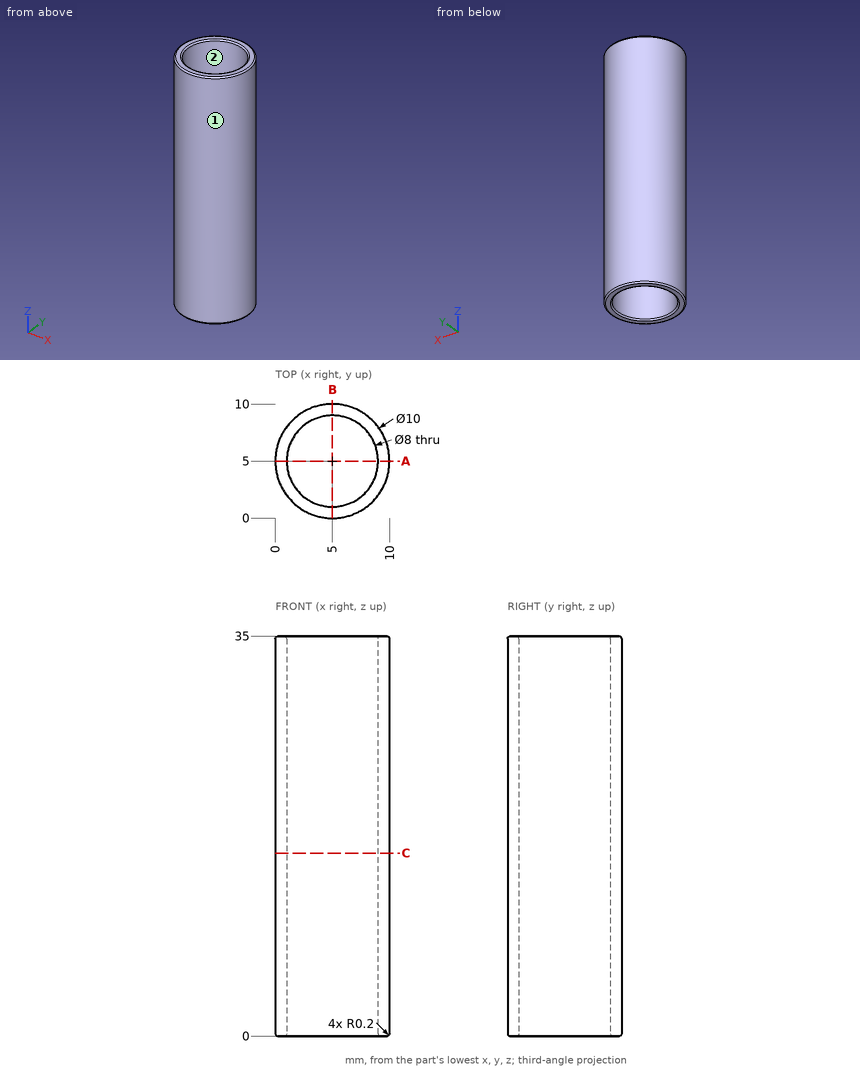
Verification items for this drawing (mm, ordinates from the low corner). Coordinates: 2 decimals unless noted, no trailing zeros. Loops run counter-clockwise (first coordinate to the right, second up) from the corner with the lowest first, then second, coordinate; pieces in that order, holes last.
Item 1: Thickness scan on line 1 (Y direction, x = 5, z = 20.5); line 2 (X direction, y = 5.25, z = 18.5); line 3 (Y direction, x = 8.5, z = 6). Record the ranges inside material, lowest first.
Item 2: Go/stop test with flat-tipped pins: pin 1 Ø6 at (x, y) = (6.5, 9) entering from -Z; pin 2 Ø3 at (x, z) = (2.5, 5.5) entering from -Y; pin 3 Ø1.5 at (y, z) = (7.5, 30) entering from -X; pin 4 Ø1 at (x, z) = (9, 8) entering from -Y. Record where each tip stops, or that it passes through.
Item 3: Sectioned sample at A-A, the plane y = 5. Record the boundary of the cut face in (x, z), then the cut area to 3 significant figures.
Item 4: Sectioned sample at C-C, the plane z = 16. Record the boundary of the cut face in (x, y), then the cut area to 3 significant figures.
Item 5: Release check for a two-part mould opening along Y. For the marked faces 1 and 2 record: released by +Y, released by -Y, zero draft, split by the parting line, or undercut.
Check result:
1. line 1: y = 0 to 1, 9 to 10
1. line 2: x = 0.01 to 1.01, 8.99 to 9.99
1. line 3: y = 1.43 to 3.06, 6.94 to 8.57
2. pin 1: stops at z = 0
2. pin 2: stops at y = 0.1
2. pin 3: stops at x = 0.32
2. pin 4: stops at y = 1.43
3. outline: (0, 0.2) arc R0.2 ccw to (0.2, 0) - (0.8, 0) arc R0.2 ccw to (1, 0.2) - (1, 34.8) arc R0.2 ccw to (0.8, 35) - (0.2, 35) arc R0.2 ccw to (0, 34.8) - close; (9, 0.2) arc R0.2 ccw to (9.2, 0) - (9.8, 0) arc R0.2 ccw to (10, 0.2) - (10, 34.8) arc R0.2 ccw to (9.8, 35) - (9.2, 35) arc R0.2 ccw to (9, 34.8) - close
3. area: 69.9 mm2
4. outline: circle Ø10 at (5, 5); hole circle Ø8 at (5, 5)
4. area: 28.3 mm2
5. face 1: split by the parting line
5. face 2: undercut
